Design review of the part built by this model. Coordinates are the model's own, in mm. Coordinates: 2 decimals unless noted, no trailing zeros. Order: outer loops, then holes, each group sorted by start corner. A loop starts at its lowest first (then second) coordinate and runs counter-clockwise, first axis right, second up. Notation, with made-up numbers: M -11.75,31 L -7.75,31 A9 cw -7.75,48 Z; hole C 80.5,25 d1. An arc over 180 degrees is marked long. Answer as a JSON object with one key per item and string values.
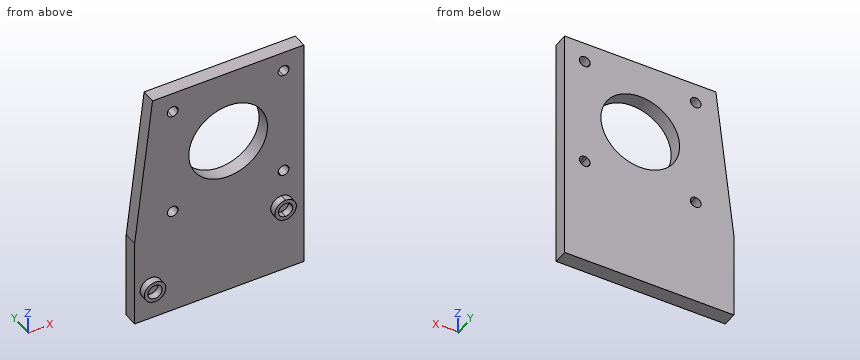
from build123d import *

# Parameters (mm, degrees)
F0_R     = 3
F0_R_2   = 11
F0_R_3   = 2
F1_DEPTH = 4
F2_DEPTH = 2


# Not quite as in the source:
# - a feature names something its author has since deleted; it is built from what else it names


with BuildPart() as f1:
    # F0 (on Front) → F1 (new body)
    with BuildSketch(Plane.XZ):
        Polygon((14.9, -21.15), (21.15, -21.15), (21.15, 21.15), (5.15, 21.15), (-21.15, 21.15), (-21.15, -21.15), align=None)
        with BuildLine():
            ThreePointArc((17, -15.5), (16.3215838363, -16.7549900398), (14.9, -16.8747727085))
            ThreePointArc((14.9, -16.8747727085), (14.2450099602, -16.3215838363), (14, -15.5))
            Line((14, -15.5), (-14, -15.5))
            ThreePointArc((-14, -15.5), (-16.5606601718, -16.5606601718), (-15.5, -14))
            Line((-15.5, -14), (-15.5, 14))
            ThreePointArc((-15.5, 14), (-16.5606601718, 16.5606601718), (-14, 15.5))
            Line((-14, 15.5), (14, 15.5))
            ThreePointArc((14, 15.5), (15.5, 17), (17, 15.5))
            ThreePointArc((17, 15.5), (16.5606601718, 14.4393398282), (15.5, 14))
            Line((15.5, 14), (15.5, -14))
            ThreePointArc((15.5, -14), (16.5606601718, -14.4393398282), (17, -15.5))
        make_face(mode=Mode.SUBTRACT)
        Polygon((21.15, -46.15), (21.15, -21.15), (14.9, -21.15), (-21.15, -21.15), (-26.15, -21.15), (-26.15, -41.15), (-26.15, -46.15), (-21.15, -46.15), align=None)
        with Locations((-21.6, -36.65)):
            Circle(F0_R, mode=Mode.SUBTRACT)
        with BuildLine():
            ThreePointArc((14.9, -29.15), (11.9, -26.15), (14.9, -23.15))
            ThreePointArc((14.9, -23.15), (17.0213203436, -24.0286796564), (17.9, -26.15))
            ThreePointArc((17.9, -26.15), (17.0213203436, -28.2713203436), (14.9, -29.15))
        make_face(mode=Mode.SUBTRACT)
        with BuildLine():
            Line((-14, -15.5), (14, -15.5))
            ThreePointArc((14, -15.5), (14.2450099602, -14.6784161637), (14.9, -14.1252272915))
            ThreePointArc((14.9, -14.1252272915), (15.1935355345, -14.0316405306), (15.5, -14))
            Line((15.5, -14), (15.5, 14))
            ThreePointArc((15.5, 14), (14.4393398282, 14.4393398282), (14, 15.5))
            Line((14, 15.5), (-14, 15.5))
            ThreePointArc((-14, 15.5), (-14.4393398282, 14.4393398282), (-15.5, 14))
            Line((-15.5, 14), (-15.5, -14))
            ThreePointArc((-15.5, -14), (-14.4393398282, -14.4393398282), (-14, -15.5))
        make_face()
        Circle(F0_R_2, mode=Mode.SUBTRACT)
        Polygon((-26.15, -21.15), (-21.15, -21.15), (-21.15, 21.15), align=None)
        with Locations((-21.6, -36.65)):
            Circle(F0_R)
        with Locations((-21.6, -36.65)):
            Circle(F0_R_3, mode=Mode.SUBTRACT)
        with Locations((-21.6, -36.65)):
            Circle(F0_R_3)
        with BuildLine():
            ThreePointArc((17.9, -26.15), (17.0213203436, -24.0286796564), (14.9, -23.15))
            Line((14.9, -23.15), (14.9, -24.15))
            ThreePointArc((14.9, -24.15), (16.3142135624, -24.7357864376), (16.9, -26.15))
            ThreePointArc((16.9, -26.15), (16.3142135624, -27.5642135624), (14.9, -28.15))
            Line((14.9, -28.15), (14.9, -29.15))
            ThreePointArc((14.9, -29.15), (17.0213203436, -28.2713203436), (17.9, -26.15))
        make_face()
        with BuildLine():
            Line((14.9, -24.15), (14.9, -23.15))
            ThreePointArc((14.9, -23.15), (11.9, -26.15), (14.9, -29.15))
            Line((14.9, -29.15), (14.9, -28.15))
            ThreePointArc((14.9, -28.15), (12.9, -26.15), (14.9, -24.15))
        make_face()
        with BuildLine():
            ThreePointArc((16.9, -26.15), (16.3142135624, -24.7357864376), (14.9, -24.15))
            Line((14.9, -24.15), (14.9, -26.15))
            Line((14.9, -26.15), (14.9, -28.15))
            ThreePointArc((14.9, -28.15), (16.3142135624, -27.5642135624), (16.9, -26.15))
        make_face()
        with BuildLine():
            Line((14.9, -26.15), (14.9, -24.15))
            ThreePointArc((14.9, -24.15), (12.9, -26.15), (14.9, -28.15))
            Line((14.9, -28.15), (14.9, -26.15))
        make_face()
    extrude(amount=-F1_DEPTH)

    # F0 (on Front) → F2 (join)
    with BuildSketch(Plane.XZ):
        with BuildLine():
            Line((14.9, -24.15), (14.9, -23.15))
            ThreePointArc((14.9, -23.15), (11.9, -26.15), (14.9, -29.15))
            Line((14.9, -29.15), (14.9, -28.15))
            ThreePointArc((14.9, -28.15), (12.9, -26.15), (14.9, -24.15))
        make_face()
        with BuildLine():
            ThreePointArc((17.9, -26.15), (17.0213203436, -24.0286796564), (14.9, -23.15))
            Line((14.9, -23.15), (14.9, -24.15))
            ThreePointArc((14.9, -24.15), (16.3142135624, -24.7357864376), (16.9, -26.15))
            ThreePointArc((16.9, -26.15), (16.3142135624, -27.5642135624), (14.9, -28.15))
            Line((14.9, -28.15), (14.9, -29.15))
            ThreePointArc((14.9, -29.15), (17.0213203436, -28.2713203436), (17.9, -26.15))
        make_face()
        with Locations((-21.6, -36.65)):
            Circle(F0_R)
        with Locations((-21.6, -36.65)):
            Circle(F0_R_3, mode=Mode.SUBTRACT)
    extrude(amount=F2_DEPTH)


solid = f1.part
1) Insertion check: pin 1 Ø8 at (x, z) = (-7.5, -32.5) entering from -Y; pin 2 Ø2.5 at (x, z) = (-15.5, -15.5) entering from -Y. Each pin has a flat end and moves straight along its axis. Give the tip position at first contact, or say it passes through.
Taken from the geometry:
{"pin 1": "stops at y = 0", "pin 2": "passes through"}
2) Add section B-B (x = 2.5). State the section outline as (y, z) points.
Taken from the geometry:
{"outline": "M 0,-46.15 L 4,-46.15 L 4,-10.71 L 0,-10.71 Z; M 0,10.71 L 4,10.71 L 4,21.15 L 0,21.15 Z"}
3) Add section A-A (y = -0.95). State the section outline as (x, z) points, and give its area (3 significant figures).
Taken from the geometry:
{"outline": "C -21.6,-36.65 d6; C 14.9,-26.15 d6; hole C -21.6,-36.65 d4; hole C 14.9,-26.15 d4", "area": "31.4 mm2"}
4) To check wall thickness, follow L1, parallel to Z at x = -15.5, y = 0.9; L2, parallel to Z at x = 0, y = 2.3; L3, parallel to X at y = 1.5, z = -15.5. State the ranges of each line that lie inside material, in increasing order.
Taken from the geometry:
{"L1": "z = -46.15 to -17, -14 to 14, 17 to 21.15", "L2": "z = -46.15 to -11, 11 to 21.15", "L3": "x = -25.48 to -17, -14 to 14, 17 to 21.15"}
5) Add section C-C (z = 2). State the section outline as (x, y) points.
Taken from the geometry:
{"outline": "M -23.41,0 L -10.82,0 L -10.82,4 L -23.41,4 Z; M 10.82,0 L 21.15,0 L 21.15,4 L 10.82,4 Z"}
6) Add section D-D (y = 2.55). State the section outline as (x, z) points.
Taken from the geometry:
{"outline": "M -26.15,-46.15 L 21.15,-46.15 L 21.15,21.15 L -21.15,21.15 L -26.15,-21.15 Z; hole C -15.5,-15.5 d3; hole C -15.5,15.5 d3; hole C 0,0 d22; hole C 15.5,-15.5 d3; hole C 15.5,15.5 d3"}
